Print and shaded views of the part. All mm, measured from the part's lowest x, y and z. A direction names the side the tool comes from. Coordinates: 2 decimals unless noted, no trailing zeros. Loops run counter-clockwise (first coordinate to the right, second up) from the corner with the lowest first, then second, coordinate; pieces in that order, holes last. Notation, with made-up numbers: (62, 44) -> (82, 44) arc R26 cw to (82, 76) -> close; hole circle Ø5 at (77, 9). An arc over 180 degrees is marked (long way). One line per question, with ' | ' between items. Start each with the question number.
1) 3-axis set-ups, long thin cutter, end or side, ignore diameter. For the marked faces 1, 2 and 3: which of +Z, -Z, +X, -X, +Y, -Y reach the whole face in a straight line?
2) Cut at D-D (z = 18). List the corners of the cut face in (x, y).
3) Drop flat-ended pins along their axis: pin 1 (2 mm diameter, centred on y = 1, z = 18, fed in from -X); pin 2 (11.5 mm diameter, centred on x = 25, z = 14, fed in from +Y); pin 3 (0.6 mm diameter, centred on x = 19.5, y = 8.5, fed in from +Z); pin 4 (6 mm diameter, centred on x = 27, z = 15.5, fed in from -Y). Give the stop position or say it passes through.
4) Cut at B-B (y = 1). List the corners of the cut face in (x, z).
5) Cut at C-C (x = 14). List the corners of the cut face in (y, z), plus the area to 3 significant figures.
6) Cut at A-A (z = 23.5). List the corners of the cut face in (x, y).
7) Probe L1, parallel to X at y = 1, z = 7; L2, parallel to Y at x = 4, z = 16.25; L3, parallel to Y at x = 8, z = 23.5. List the from-to ranges inside material, lowest first. Write a range as from..to.
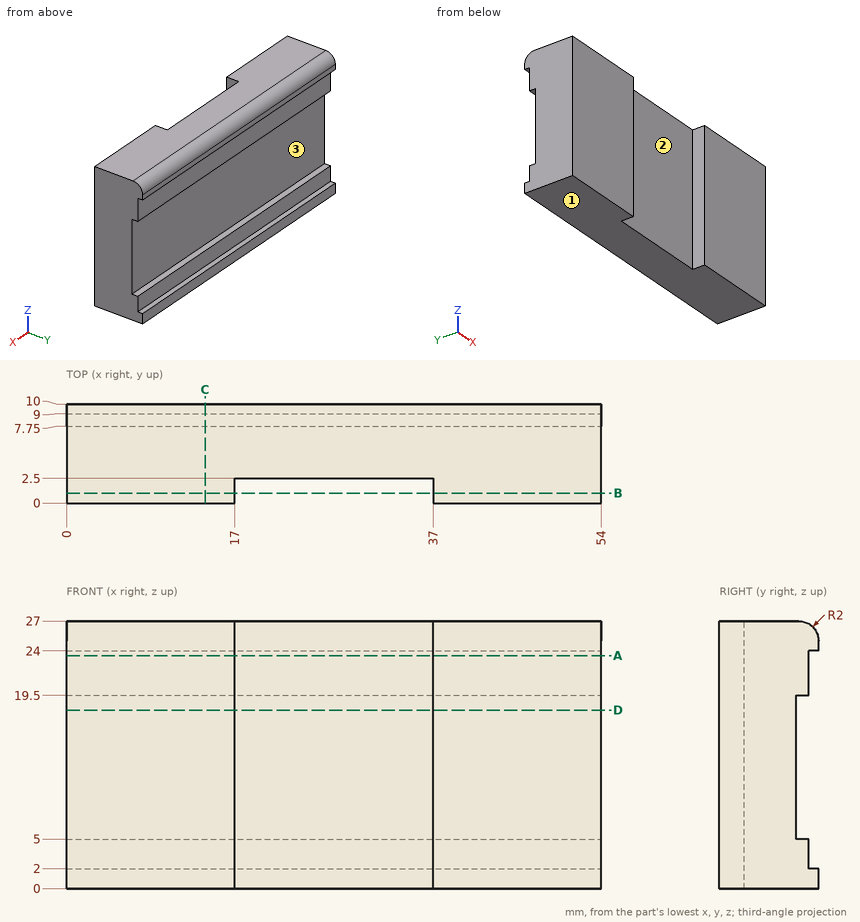
Reported:
1) face 1: -Z, +X, -X, +Y, -Y | face 2: +Z, -Z, -Y | face 3: +X, -X, +Y
2) outline: (0, 0) -> (17, 0) -> (17, 2.5) -> (37, 2.5) -> (37, 0) -> (54, 0) -> (54, 7.75) -> (0, 7.75) -> close
3) pin 1: stops at x = 0 | pin 2: stops at y = 9 | pin 3: stops at z = 26.99 | pin 4: stops at y = 2.5
4) outline: (0, 0) -> (17, 0) -> (17, 27) -> (0, 27) -> close; (37, 0) -> (54, 0) -> (54, 27) -> (37, 27) -> close
5) outline: (0, 0) -> (10, 0) -> (10, 2) -> (9, 2) -> (9, 5) -> (7.75, 5) -> (7.75, 19.5) -> (9, 19.5) -> (9, 24) -> (10, 24) -> (10, 25) arc R2 ccw to (8, 27) -> (0, 27) -> close | area: 229 mm²
6) outline: (0, 0) -> (17, 0) -> (17, 2.5) -> (37, 2.5) -> (37, 0) -> (54, 0) -> (54, 9) -> (0, 9) -> close
7) L1: x = 0..17, 37..54 | L2: y = 0..7.75 | L3: y = 0..9
